```python
from build123d import *

# Parameters (mm, degrees)
SKETCH1_R           = 10
BOSS_EXTRUDE1_DEPTH = 2
SKETCH3_R           = 2
BOSS_EXTRUDE2_DEPTH = 10
SKETCH4_R           = 2
BOSS_EXTRUDE3_DEPTH = 20


with BuildPart() as part:
    # Sketch1 → Boss-Extrude1 (new body)
    with BuildSketch(Plane.XY):
        Circle(SKETCH1_R)
    extrude(amount=BOSS_EXTRUDE1_DEPTH)

    # Sketch3 → Boss-Extrude2 (add)
    with BuildSketch(Plane(origin=(0, 0, 0), x_dir=(-1, 0, 0), z_dir=(0, -0.7071067811865476, -0.7071067811865476))):
        with Locations(Location((0, 0, 0), (0, 0, 180))):
            Circle(SKETCH3_R)
    extrude(amount=BOSS_EXTRUDE2_DEPTH)

    # Sketch4 → Boss-Extrude3 (add)
    with BuildSketch(Plane(origin=(0, 0, 0), x_dir=(-1, 0, 0), z_dir=(0, 0.7071067811865477, -0.7071067811865475))):
        Circle(SKETCH4_R)
    extrude(amount=BOSS_EXTRUDE3_DEPTH)


solid = part.part
```
Build history of the part. All positions in model axes, mm. Coordinates: 2 decimals unless noted, no trailing zeros. Order: outer loops, then holes, each group sorted by start corner. A loop starts at its lowest first (then second) coordinate and runs counter-clockwise, first axis right, second up.
Item 1: Mould opens along Z. For faces 1 (the cylindrical face through (-2, -4, -4)), 2 (the cylindrical face through (-2.17, -9.76, 0.99)), 3 (the flat face through (-0.03, -7.09, -7.05)), 4 (the cylindrical face through (-2, 7, -7)) say: released by +Z, released by -Z, zero draft, split by the parting line, or undercut.
Filled in:
face 1: undercut
face 2: zero draft
face 3: released by -Z
face 4: undercut
Item 2: Drill centre lines: L1, parallel to Z at x = -7.5, y = 2; L2, parallel to Y at x = -0.25, z = -7.5; L3, parallel to Z at x = -1, y = -4.25. Where is each one in solid material? Low to high.
Filled in:
L1: z = 0 to 2
L2: y = -6.64 to -4.69, 4.69 to 10.31
L3: z = -6.7 to -1.8, 0 to 2
Item 3: Saw through at B-B on x = -8. List the corners of the cut face in (y, z), then the cut area to 3 significant figures.
Filled in:
outline: (-6, 0) - (6, 0) - (6, 2) - (-6, 2) - close
area: 24.0 mm2
Item 4: Saw through at C-C on x = 7. List the corners of the cut face in (y, z).
Filled in:
outline: (-7.14, 0) - (7.14, 0) - (7.14, 2) - (-7.14, 2) - close
Item 5: Saw through at A-A on x = 1.25. List the corners of the cut face in (y, z), then the cut area to 3 significant figures.
Filled in:
outline: (-9.92, 0) - (-2.21, 0) - (-8.18, -5.97) - (-5.97, -8.18) - (0, -2.21) - (13.04, -15.25) - (15.25, -13.04) - (2.21, 0) - (9.92, 0) - (9.92, 2) - (-9.92, 2) - close
area: 128 mm2
Item 6: Drop flat-ended pins along their axis: pin 1 Ø2 at (x, z) = (-3.5, -0.5) entering from +Y; pin 2 Ø1.5 at (y, z) = (5, -10) entering from -X; pin 3 Ø6 at (x, y) = (4, -4) entering from -Z; pin 4 Ø8 at (x, z) = (2.5, -5) entering from +Y. Give the stop position or say it passes through.
Filled in:
pin 1: stops at y = 9.65
pin 2: passes through
pin 3: stops at z = -7.53
pin 4: stops at y = 11.22
